from build123d import *

# Parameters (mm, degrees)
TUBE_R         = 25
TUBE_R_2       = 21
TUBE_DEPTH     = 20
FILLET_R       = 2
CYLINDER_R     = 25
CYLINDER_DEPTH = 10


with BuildPart() as fillet_body:
    # Tube → Tube (new body)
    with BuildSketch(Plane.XY.offset(10)):
        Circle(TUBE_R)
        Circle(TUBE_R_2, mode=Mode.SUBTRACT)
    extrude(amount=TUBE_DEPTH)

    # Fillet
    fillet_edges = [fillet_body.edges().sort_by_distance(p)[0] for p in [
        (-21, 0, 30),
    ]]
    fillet(fillet_edges, radius=FILLET_R)


with BuildPart() as fusion:
    # Cylinder → Cylinder (new body)
    with BuildSketch(Plane.XY):
        Circle(CYLINDER_R)
    extrude(amount=CYLINDER_DEPTH)

    # Fusion: union Fillet body
    add(fillet_body.part)


solid = fusion.part
Source: CAD feature listing. Evaluate the final solid. Frame: model axes, mm. A direction names the side the tool comes from. Coordinates: 2 decimals unless noted, no trailing zeros. Write each loop counter-clockwise with the first axis right and the second up, starting at its lowest first coordinate (ties: lowest second). Pieces come first, ordered by that corner, then holes. Notation, with made-up numbers: M -19,-15 L 32,-15 A28 ccw 32,5 Z; hole C 31,39 d1. An arc over 180 degrees is marked long. Use a Markdown table: item, result.
1) First-contact query: pin 1 Ø4 at (y, z) = (-15.5, 25) entering from +X; pin 2 Ø6 at (x, z) = (3, 9.5) entering from +Y; pin 3 Ø1.5 at (x, z) = (8.5, 16) entering from -Y. Flat tips, straight axial feed; report the tip coordinate or a pass-through.
Conclusion:
| item | result |
|---|---|
| pin 1 | stops at x = 21.04 |
| pin 2 | stops at y = 25 |
| pin 3 | stops at y = -23.77 |
2) Mould query, pull axis X, two halves, no side actions, for faces 3 (the flat face through (22.1, -7.3, 30)), 4 (the cylindrical face through (20.03, 6.31, 18.87)), 5 (the cylindrical face through (23.846, 7.509, 14.79)). Classes: pulls with the +X half, pulls with the -X half, needs draft (parallel to the pull), parting line crosses it, or undercut.
Conclusion:
| item | result |
|---|---|
| face 3 | needs draft |
| face 4 | undercut |
| face 5 | parting line crosses it |
3) Section D-D, the plane z = 7.75. Output: boundary loops of the cut face in (x, y).
Conclusion:
| item | result |
|---|---|
| outline | C 0,0 d50 |
4) Reachability of faces 1 (the flat face through (0, 0, 0)), 2 (the flat face through (0, 0, 10)) from +Z, -Z, +X, -X, +Y, -Y: full face, straight path, thin tool, end or side. Return the list, or none.
Conclusion:
| item | result |
|---|---|
| face 1 | -Z, +X, -X, +Y, -Y |
| face 2 | +Z |
5) Ray query, L1, parallel to Y at x = 0, z = 21; L2, parallel to Z at x = 5, y = 1; L3, parallel to X at y = -3, z = 15.5. Return the intervals inside material, ascending.
Conclusion:
| item | result |
|---|---|
| L1 | y = -25 to -21, 21 to 25 |
| L2 | z = 0 to 10 |
| L3 | x = -24.82 to -20.78, 20.78 to 24.82 |
6) Section B-B, the plane z = 15.5. Output: boundary loops of the cut face in (x, y).
Conclusion:
| item | result |
|---|---|
| outline | C 0,0 d50; hole C 0,0 d42 |
7) Section A-A, the plane y = 0. Output: boundary loops of the cut face in (x, z).
Conclusion:
| item | result |
|---|---|
| outline | M -25,0 L 25,0 L 25,30 L 23,30 A2 ccw 21,28 L 21,10 L -21,10 L -21,28 A2 ccw -23,30 L -25,30 Z |
